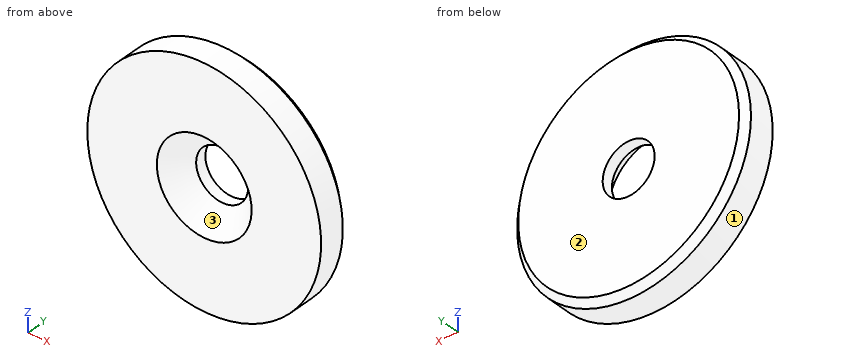
Autodesk Inventor part; units mm, degrees
ref_plane "YZ Plane" through (0, 0, 0) normal (1, 0, 0) x (0, 1, 0)
ref_plane "XZ Plane" through (0, 0, 0) normal (0, 1, 0) x (-1, 0, 0)
ref_plane "XY Plane" through (0, 0, 0) normal (0, 0, 1) x (1, 0, 0)
sketch "Boceto1" plane through (0, 0, 0) normal (0, 1, 0) x (-1, 0, 0)
  circle A0 centre (0, 0) radius 9
  dimension "d0" = 18
extrude "Extrusión1" add sketch "Boceto1" along normal blind 2.5
chamfer "Chaflán1" distance 0.5 angle 45 1 edges at (9, 2.5, 0)
sketch "Boceto2" plane through (0, 0, 0) normal (0, -1, 0) x (1, 0, 0)
  circle A0 centre (0, 0) radius 8.5
  line L0 (9, 0) -> (0, 0)
hole "Agujero1" at (0, 0, 0) direction (0, 1, 0) diameter 4 end through all countersink diameter 7.3 countersink angle 90
properties part number "markers_base2"
Verification items for the finished model (mm, model axes). Face numbers are marked on the shaded views. Give positions to 0.01 mm unless a question says otherwise; leave off trailing zeros. Order: outer loops, then holes, each group sorted by start corner. A loop starts at its lowest first (then second) coordinate and runs counter-clockwise, first axis right, second up. Notation, with made-up numbers: M 71.25,72.25 L 110.25,72.25 A9 cw 110.25,78.25 Z; hole C 15,14 d6. An arc over 180 degrees is marked long. Answer in a Markdown table with one row per item. Add a question column.
Item 1: Gauge pin test, flat end, axial feed: pin 1 (1.5 mm diameter, centred on y = 0.5, z = -4, fed in from -X). Record the tip position at first contact, or that the pin passes through.
Item 2: Mould release check, pull along X, two halves, no side actions. Record for the marked faces 1, 2 and 3: released by +X, released by -X, zero draft, split by the parting line, or undercut.
Item 3: Section check D-D, the plane y = 2.25. Enter the section's corners in (x, z), and give its area (3 significant figures).
Item 4: Scan lines: probe 1 along Z at (x, y) = (0, 2.1); probe 2 along Z at (x, y) = (0, 1.9); probe 3 along X at (y, z) = (0.9, -0.5). Record each from-to range of solid material in increasing order. Write a range as from..to.
Item 5: Section check A-A, the plane x = 0. Enter the section's corners in (y, z).
Item 6: Section check B-B, the plane z = 0. Enter the section's corners in (x, y).
Item 7: Section check C-C, the plane y = 1.05. Enter the section's corners in (x, z), and give its area (3 significant figures).
Filled sheet:
| question | item | result |
|---|---|---|
| 1 | pin 1 | stops at x = -8.39 |
| 2 | face 1 | split by the parting line |
| 2 | face 2 | zero draft |
| 2 | face 3 | undercut |
| 3 | outline | C 0,0 d17.5; hole C 0,0 d4 |
| 3 | area | 228 mm^2 |
| 4 | probe 1 | z = -8.9..-2, 2..8.9 |
| 4 | probe 2 | z = -9..-2, 2..9 |
| 4 | probe 3 | x = -8.99..-2.7, 2.7..8.99 |
| 5 | outline | M 0,-9 L 2,-9 L 2.5,-8.5 L 2.5,-2 L 1.65,-2 L 0,-3.65 Z; M 0,3.65 L 1.65,2 L 2.5,2 L 2.5,8.5 L 2,9 L 0,9 Z |
| 6 | outline | M -9,0 L -3.65,0 L -2,1.65 L -2,2.5 L -8.5,2.5 L -9,2 Z; M 2,1.65 L 3.65,0 L 9,0 L 9,2 L 8.5,2.5 L 2,2.5 Z |
| 7 | outline | C 0,0 d18; hole C 0,0 d5.2 |
| 7 | area | 233 mm^2 |
